Here's how the part is built. I have some questions about the finished solid (model axes, mm). Face numbers are marked on the shaded views. A direction names the side the tool comes from. Coordinates: 2 decimals unless noted, no trailing zeros. Loops run counter-clockwise (first coordinate to the right, second up) from the corner with the lowest first, then second, coordinate; pieces in that order, holes last. Notation, with made-up numbers: (67.5, -19.5) -> (92.5, -19.5) arc R25 ccw to (92.5, 10.5) -> close; hole circle Ø4 at (72.25, -13.5). An arc over 180 degrees is marked (long way). Answer as a JSON object with one key per item and string values. Group by question number.
1) I want a section at C-C (x = 39.5). Write out the boundary of the cut face in (y, z), then the cut area to 3 significant figures.
2) I need wall thicknesses on probe 1 along X at (y, z) = (-2.5, 3.45); probe 2 along Z at (x, y) = (33.25, -1.75); probe 3 along X at (y, z) = (-1.15, 15.75). Which ranges of each line are inside material? Lowest first, please. Write a range as [from, to].
3) Which directions (+Z, -Z, +X, -X, +Y, -Y) give clear straight access to the entire face, cutting with the end or side of a thin tool? Please do the marked faces 1 and 2.
4) I want a section at A-A (z = 12). Write out the boundary of the cut face in (x, y).
5) I'm going to push flat-ended pins straight in: pin 1 (2 mm diameter, centred on x = 14.5, y = -3, fed in from -Z); pin 2 (1.5 mm diameter, centred on x = 21.5, y = -3, fed in from -Z); pin 3 (2.5 mm diameter, centred on x = 35, y = -2.5, fed in from +Z); pin 4 (13 mm diameter, centred on x = 10.75, z = 12, fed in from +Y). Where does each tip first touch, or does it pass through?
6) I want a section at D-D (z = 8.5). Write out the boundary of the cut face in (x, y).
7) I want a section at B-B (x = 31.5). Write out the boundary of the cut face in (y, z).
8) If we mould it in two halves opening along X, with no side actions, what happens to the marked faces 3, 4 and 5? For each: +X half, -X half, draft (parallel to the pull), parting line (faces both ways), or undercut.
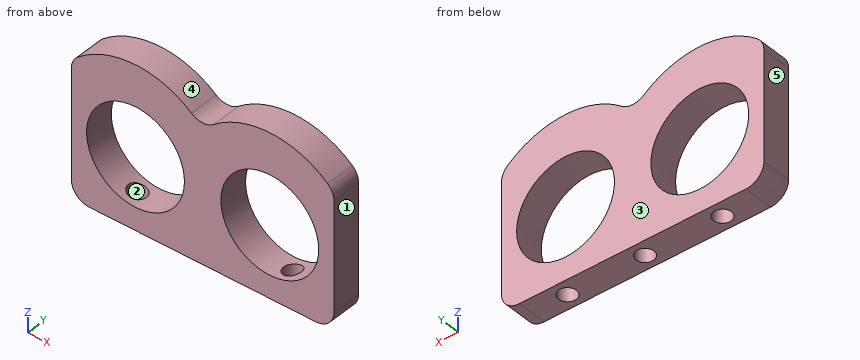
```python
from build123d import *

# Parameters (mm, degrees)
SKETCH_R     = 8.2
PAD_DEPTH    = 5
FILLET_R     = 3
FILLET001_R  = 3
FILLET002_R  = 3
SKETCH001_R  = 1.5
POCKET_DEPTH = 5


with BuildPart() as part:
    # Sketch → Pad (new body)
    with BuildSketch(Plane.XZ):
        with BuildLine():
            Line((0, 0), (44, 0))
            Line((44, 0), (44, 22.535654))
            ThreePointArc((44, 22.535654), (32.883624, 27.047534), (22, 22))
            ThreePointArc((22, 22), (11.116376, 27.047534), (0, 22.535654))
            Line((0, 0), (0, 22.535654))
        make_face()
        with Locations((10.75, 12)):
            Circle(SKETCH_R, mode=Mode.SUBTRACT)
        with Locations((33.25, 12)):
            Circle(SKETCH_R, mode=Mode.SUBTRACT)
    extrude(amount=PAD_DEPTH)

    # Fillet
    fillet_edges = [part.edges().sort_by_distance(p)[0] for p in [
        (0, -2.5, 0),
        (44, -2.5, 0),
    ]]
    fillet(fillet_edges, radius=FILLET_R)

    # Fillet001
    fillet001_edges = [part.edges().sort_by_distance(p)[0] for p in [
        (22, -2.5, 22),
    ]]
    fillet(fillet001_edges, radius=FILLET001_R)

    # Fillet002
    fillet002_edges = [part.edges().sort_by_distance(p)[0] for p in [
        (44, -2.5, 22.535654),
        (0, -2.5, 22.535654),
    ]]
    fillet(fillet002_edges, radius=FILLET002_R)

    # Sketch001 → Pocket (cut)
    with BuildSketch(Plane(origin=(0, 0, 0), x_dir=(1, 0, 0), z_dir=(0, 0, -1))):
        with Locations((9, 2.5)):
            Circle(SKETCH001_R)
        with Locations((35, 2.5)):
            Circle(SKETCH001_R)
        with Locations((22, 2.5)):
            Circle(SKETCH001_R)
    extrude(amount=-POCKET_DEPTH, mode=Mode.SUBTRACT)


solid = part.part
```
Determined:
{
 "1": {"outline": "(-5, 0) -> (0, 0) -> (0, 6.69) -> (-5, 6.69) -> close; (-5, 17.31) -> (0, 17.31) -> (0, 25.69) -> (-5, 25.69) -> close", "area": "75.4 mm^2"},
 "2": {"probe 1": "[0, 7.5], [10.5, 20.5], [23.5, 33.5], [36.5, 44]", "probe 2": "[0, 3.8], [20.2, 27.05]", "probe 3": "[0, 3.46], [18.04, 25.96], [40.54, 44]"},
 "3": {"face 1": "+Z, -Z, +X, +Y, -Y", "face 2": "-Z"},
 "4": {"outline": "(0, -5) -> (2.55, -5) -> (2.55, 0) -> (0, 0) -> close; (18.95, -5) -> (25.05, -5) -> (25.05, 0) -> (18.95, 0) -> close; (41.45, -5) -> (44, -5) -> (44, 0) -> (41.45, 0) -> close"},
 "5": {"pin 1": "z = 0", "pin 2": "z = 5", "pin 3": "z = 27.04", "pin 4": "through"},
 "6": {"outline": "(0, -5) -> (3.33, -5) -> (3.33, 0) -> (0, 0) -> close; (18.17, -5) -> (25.83, -5) -> (25.83, 0) -> (18.17, 0) -> close; (40.67, -5) -> (44, -5) -> (44, 0) -> (40.67, 0) -> close"},
 "7": {"outline": "(-5, 0) -> (0, 0) -> (0, 3.99) -> (-5, 3.99) -> close; (-5, 20.01) -> (0, 20.01) -> (0, 26.95) -> (-5, 26.95) -> close"},
 "8": {"face 3": "draft", "face 4": "undercut", "face 5": "-X half"}
}
